Here's the drawing with two shaded views (mm, measured from the low corner). I have some questions. A direction names the side the tool comes from. Coordinates: 2 decimals unless noted, no trailing zeros. Write each loop counter-clockwise with the first axis right and the second up, starting at its lowest first coordinate (ties: lowest second). Pieces come first, ordered by that corner, then holes. Notation, with made-up numbers: M 27,75 L 83,75 A23 ccw 83,87 Z; hole C 59.5,50.5 d1. An arc over 180 degrees is marked long. Use one line per item in the form item = value. Start each with the question number.
1. I want a section at A-A, the plane z = 7.3. List the corners of the cut face in (x, y) for me, plus the area to 3 significant figures.
2. Please list where these lines run through material, in increasing order: line 1 along X through (y, z) = (17.5, 7.3); line 2 along X through (y, z) = (17.25, 7.3). Write a range as [from, to].
3. On a 3-axis mill with a long thin cutter (end or side, diameter ignored), from which of +Z, -Z, +X, -X, +Y, -Y can I reach the whole of each face in a straight line? I mean the marked faces 1, 2, 3, 4 and 5. Say none if no direction works.
4. I want a section at C-C, the plane y = 19.5. List the corners of the cut face in (x, z) for me.
5. I'm going to push flat-ended pins straight in: pin 1 Ø5 at (x, y) = (5.5, 13) entering from +Z; pin 2 Ø3 at (x, y) = (8, 15) entering from -Z; pin 3 Ø3 at (y, z) = (15, 7.5) entering from +X; pin 4 Ø5 at (x, z) = (5, 8) entering from -Y. Where does each tip first touch, or does it pass through?
6. I want a section at B-B, the plane x = 9. List the corners of the cut face in (y, z) for me.
7. I want a section at D-D, the plane y = 16. List the corners of the cut face in (x, z) for me, plus the area to 3 significant figures.
8. Thinking about a two-plate mould opening in X: for the marked faces 6, 7, 8 and 9, which applies, released by +X, released by -X, zero draft, split by the parting line, or undercut?
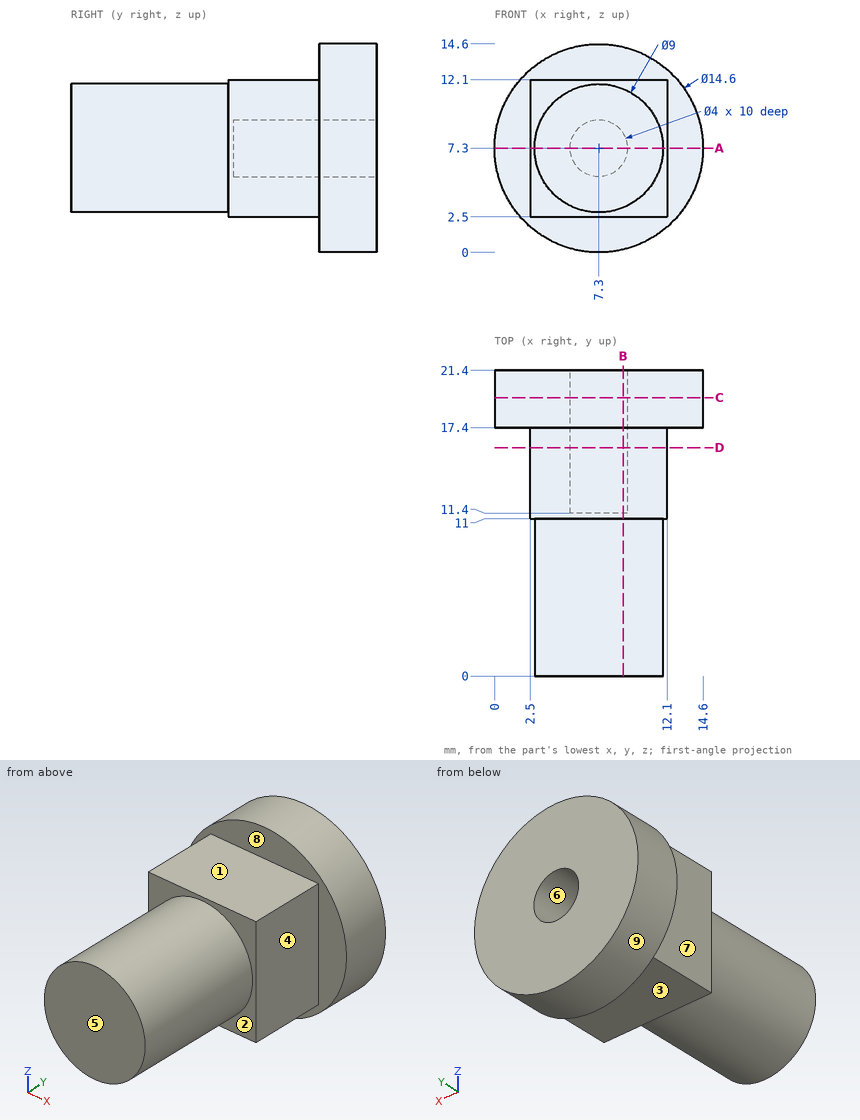
Answer list:
q1.outline = M 0,17.4 L 2.5,17.4 L 2.5,11 L 2.8,11 L 2.8,0 L 11.8,0 L 11.8,11 L 12.1,11 L 12.1,17.4 L 14.6,17.4 L 14.6,21.4 L 9.3,21.4 L 9.3,11.4 L 5.3,11.4 L 5.3,21.4 L 0,21.4 Z
q1.area = 179 mm²
q2.line_1 = [0, 5.3], [9.3, 14.6]
q2.line_2 = [2.5, 5.3], [9.3, 12.1]
q3.face_1 = +Z, +X, -X, -Y
q3.face_2 = -Y
q3.face_3 = -Z, +X, -X, -Y
q3.face_4 = +Z, -Z, +X, -Y
q3.face_5 = +Z, -Z, +X, -X, -Y
q4.outline = C 7.3,7.3 d14.6; hole C 7.3,7.3 d4
q5.pin_1 = 12.1
q5.pin_2 = 2.5
q5.pin_3 = 12.1
q5.pin_4 = 0
q6.outline = M 0,3.13 L 11,3.13 L 11,2.5 L 17.4,2.5 L 17.4,0.2 L 21.4,0.2 L 21.4,6.25 L 11.4,6.25 L 11.4,8.35 L 21.4,8.35 L 21.4,14.4 L 17.4,14.4 L 17.4,12.1 L 11,12.1 L 11,11.47 L 0,11.47 Z
q7.outline = M 2.5,2.5 L 12.1,2.5 L 12.1,12.1 L 2.5,12.1 Z; hole C 7.3,7.3 d4
q7.area = 79.6 mm²
q8.face_6 = undercut
q8.face_7 = released by -X
q8.face_8 = zero draft
q8.face_9 = split by the parting line
